Geometry: final body of the model. Coordinates: model frame, mm. Round coordinates to 2 decimals unless told otherwise and drop trailing zeros. Loops run counter-clockwise (first coordinate to the right, second up) from the corner with the lowest first, then second, coordinate; pieces in that order, holes last. Notation, with made-up numbers: M 80,7.5 L 114,7.5 A29 cw 114,37.5 Z; hole C 35,-0.5 d11. An arc over 180 degrees is marked long. Return JSON: item names as keys, results as strings.
from build123d import *

# Parameters (mm, degrees)
SKETCH2_R          = 1.65
CUT_EXTRUDE1_DEPTH = 6
FILLET1_R          = 0.25


with BuildPart() as part:
    # Sketch1 → Revolve1 (revolve)
    with BuildSketch(Plane.XY, mode=Mode.PRIVATE) as revolve1_sk:
        with BuildLine():
            Line((0, 3), (2, 3))
            Line((2, 3), (2, 2.1))
            ThreePointArc((2, 2.1), (2.9, 0), (2, -2.1))
            Line((2, -2.1), (2, -3))
            Line((2, -3), (0, -3))
            Line((0, -3), (0, 3))
        make_face()
    revolve(revolve1_sk.sketch.rotate(Axis((0, 4.183554313, 0), (0, -1, 0)), 90), axis=Axis((0, 4.183554313, 0), (0, -1, 0)))

    # Sketch2 → Cut-Extrude1 (cut)
    with BuildSketch(Plane(origin=(0, 3, 0), x_dir=(1, 0, 0), z_dir=(0, 1, 0))):
        with Locations(Location((0, 0, 0), (0, 0, 270))):
            Circle(SKETCH2_R)
    extrude(amount=-CUT_EXTRUDE1_DEPTH, mode=Mode.SUBTRACT)

    # Fillet1
    fillet1_edges = [part.edges().sort_by_distance(p)[0] for p in [
        (0, -2.1, -2),
        (0, 2.1, -2),
    ]]
    fillet(fillet1_edges, radius=FILLET1_R)


solid = part.part
Q1. Material intervals for L1, parallel to Z at x = 1.5, y = 2.5; L2, parallel to X at y = 1.5, z = 0.65; L3, parallel to Z at x = -1, y = -1.25, sorted ascending.
Determined:
{"L1": "z = -1.32 to -0.69, 0.69 to 1.32", "L2": "x = -2.4 to -1.52, 1.52 to 2.4", "L3": "z = -2.42 to -1.31, 1.31 to 2.42"}
Q2. Section query C-C (y = 1.25). Output: boundary loops of the cut face in (x, z).
Determined:
{"outline": "C 0,0 d5.23; hole C 0,0 d3.3"}
Q3. Section query A-A (y = -0.25). Output: boundary loops of the cut face in (x, z), plus the area to 3 significant figures.
Determined:
{"outline": "C 0,0 d5.78; hole C 0,0 d3.3", "area": "17.7 mm^2"}
Q4. Pin query (flat end, axial travel): pin 1 (1 mm diameter, centred on y = -0.5, z = -2, fed in from -X). Return the tip coordinate at first contact, or that it passes through.
Determined:
{"pin 1": "stops at x = -2.44"}
Q5. Pull-direction query (X, two-part tool) for faces 1 (the cylindrical face through (0.766, -2.608, 1.847)), 2 (the cylindrical face through (-1, 0.04, -1.31)); classes: pulls with the +X half, pulls with the -X half, needs draft (parallel to the pull), parting line crosses it, or undercut.
Determined:
{"face 1": "parting line crosses it", "face 2": "undercut"}
Q6. Section query B-B (x = -2.4). Output: boundary loops of the cut face in (y, z), plus the area to 3 significant figures.
Determined:
{"outline": "C 0,0 d3.26", "area": "8.33 mm^2"}
